from build123d import *

# Parameters (mm, degrees)
ESQUISSE1_R             = 38.5
BOSS_EXTRU_1_DEPTH      = 100
ENL_V_START             = -95
ESQUISSE2_R             = 38.5
ESQUISSE2_R_2           = 28.5
ENL_V_MAT_EXTRU_1_DEPTH = 95
ESQUISSE4_R             = 22.5
ENL_V_MAT_EXTRU_2_DEPTH = 45
ESQUISSE5_R             = 18.5
ENL_V_MAT_EXTRU_3_DEPTH = 9
ESQUISSE6_R             = 12
ENL_V_MAT_EXTRU_4_DEPTH = 77.684418235
D_GAGEMENT_M222_D       = 24
ESQUISSE14_R            = 1.5
ENL_V_MAT_EXTRU_8_DEPTH = 77.684418235
ENL_V_START_2           = -9
ESQUISSE16_R            = 18.5
ENL_V_MAT_EXTRU_9_DEPTH = 9


with BuildPart() as part:
    # Esquisse1 → Boss.-Extru.1 (new body)
    with BuildSketch(Plane(origin=(0, 0, 0), x_dir=(1, 0, 0), z_dir=(0, 1, 0))):
        with Locations(Location((0, 0, 0), (0, 0, 270))):
            Circle(ESQUISSE1_R)
    extrude(amount=BOSS_EXTRU_1_DEPTH)

    # Esquisse2 → Enlèv. mat.-Extru.1 (cut)
    with BuildSketch(Plane(origin=(0, 100, 0), x_dir=(1, 0, 0), z_dir=(0, 1, 0)).offset(ENL_V_START)):
        with Locations(Location((0, 0, 0), (0, 0, 270))):
            Circle(ESQUISSE2_R)
        with Locations(Location((0, 0, 0), (0, 0, 270))):
            Circle(ESQUISSE2_R_2, mode=Mode.SUBTRACT)
    extrude(amount=ENL_V_MAT_EXTRU_1_DEPTH, mode=Mode.SUBTRACT)

    # Esquisse4 → Enlèv. mat.-Extru.2 (cut)
    with BuildSketch(Plane(origin=(0, 0, 0), x_dir=(-1, 0, 0), z_dir=(0, -1, 0))):
        with Locations(Location((0, 0, 0), (0, 0, 90))):
            Circle(ESQUISSE4_R)
    extrude(amount=-ENL_V_MAT_EXTRU_2_DEPTH, mode=Mode.SUBTRACT)

    # Esquisse5 → Enlèv. mat.-Extru.3 (cut)
    with BuildSketch(Plane(origin=(0, 45, 0), x_dir=(-1, 0, 0), z_dir=(0, -1, 0))):
        with Locations(Location((0, 0, 0), (0, 0, 90))):
            Circle(ESQUISSE5_R)
    extrude(amount=-ENL_V_MAT_EXTRU_3_DEPTH, mode=Mode.SUBTRACT)

    # Esquisse6 → Enlèv. mat.-Extru.4 (cut, through all)
    with BuildSketch(Plane(origin=(0, 54, 0), x_dir=(-1, 0, 0), z_dir=(0, -1, 0))):
        with Locations(Location((0, 0, 0), (0, 0, 90))):
            Circle(ESQUISSE6_R)
    extrude(amount=-ENL_V_MAT_EXTRU_4_DEPTH, mode=Mode.SUBTRACT)

    # Dégagement M222 (through all)
    with Locations(Plane(origin=(0, 72.5, 28.5), x_dir=(1, 0, 0), z_dir=(0, 0, 1))):
        with Locations((0, 0)):
            Hole(D_GAGEMENT_M222_D / 2)

    # Esquisse14 → Enlèv. mat.-Extru.8 (cut, through all)
    with BuildSketch(Plane(origin=(0, 54, 0), x_dir=(-1, 0, 0), z_dir=(0, -1, 0))):
        with Locations(Location((0, -33.5, 0), (0, 0, 270))):
            Circle(ESQUISSE14_R)
        with Locations(Location((-29.011851027, -16.75, 0), (0, 0, 270))):
            Circle(ESQUISSE14_R)
        with Locations(Location((-29.011851027, 16.75, 0), (0, 0, 270))):
            Circle(ESQUISSE14_R)
        with Locations(Location((0, 33.5, 0), (0, 0, 270))):
            Circle(ESQUISSE14_R)
        with Locations(Location((29.011851027, 16.75, 0), (0, 0, 270))):
            Circle(ESQUISSE14_R)
        with Locations(Location((29.011851027, -16.75, 0), (0, 0, 270))):
            Circle(ESQUISSE14_R)
    extrude(amount=ENL_V_MAT_EXTRU_8_DEPTH, mode=Mode.SUBTRACT)

    # Esquisse16 → Enlèv. mat.-Extru.9 (cut)
    with BuildSketch(Plane(origin=(0, 100, 0), x_dir=(1, 0, 0), z_dir=(0, 1, 0)).offset(ENL_V_START_2)):
        with Locations(Location((0, 0, 0), (0, 0, 90))):
            Circle(ESQUISSE16_R)
    extrude(amount=ENL_V_MAT_EXTRU_9_DEPTH, mode=Mode.SUBTRACT)


solid = part.part
Here's how the part is built. I have some questions about the finished solid (model axes, mm). A direction names the side the tool comes from. Coordinates: 2 decimals unless noted, no trailing zeros. Order: outer loops, then holes, each group sorted by start corner. A loop starts at its lowest first (then second) coordinate and runs counter-clockwise, first axis right, second up. Notation, with made-up numbers: M -11,87 L -4,87 A9 cw -4,93 Z; hole C 79,-15.5 d4. An arc over 180 degrees is marked long. Answer as CSV lines item,"result". Start each with the question number.
1. For pin 1 (4 mm diameter, centred on x = 29.01, z = -16.75, fed in from -Y); pin 2 (1 mm diameter, centred on y = 32.5, z = 5, fed in from +X); pin 3 (3 mm diameter, centred on x = 22, y = 62, fed in from +Z); pin 4 (4 mm diameter, centred on y = 67, z = -9.5, fed in from -X), each with a flat end and sliding along its axis, tell me the tip position at first contact or that it passes through.
2. I want a section at C-C, the plane z = -6.5. Write out the boundary of the cut face in (x, y), and give its area (3 significant figures).
3. I want a section at A-A, the plane z = -16.75. Count the separate pieces of the cut face and the enclosed holes in it, and give its area (3 significant figures).
4. On a 3-axis mill with a long thin cutter (end or side, diameter ignored), from which of +Z, -Z, +X, -X, +Y, -Y can I reach the whole of each face in a straight line? I mean faces 5 (the flat face through (29, 5, 0)), 6 (the cylindrical face through (11.9, 85.73, 1.56)), 7 (the flat face through (-18, 45, 5)). Say none if no direction works.
5. We'd pull the mould along X, two halves only. Please class faces 1 (the cylindrical face through (7.086, 95.437, -17.089)), 2 (the cylindrical face through (-37.584, 2.465, -8.346)), 3 (the cylindrical face through (30.476, 2.535, -17.075)), 4 (the flat face through (-17, 0, 17)): released by +X, released by -X, zero draft, split by the parting line, or undercut.
6. I need wall thicknesses on line 1 (Y direction, x = -30.5, z = 5.5); line 2 (Y direction, x = -3, z = 18.5); line 3 (X direction, y = 54.5, z = -2.5). Which ranges of each line are inside material? Lowest first, please. Write a range as [from, to].
7. I want a section at B-B, the plane y = 64. Write out the boundary of the cut face in (x, z), and give its area (3 significant figures).
Recorded:
1,pin 1,"stops at y = 0"
1,pin 2,"stops at x = 28.14"
1,pin 3,"stops at z = 19.8"
1,pin 4,"stops at x = -27.5"
2,outline,"M -37.95,0 L -21.54,0 L -21.54,45 L -17.32,45 L -17.32,54 L -10.09,54 L -10.09,66 A12 cw -10.09,79 L -10.09,91 L -17.32,91 L -17.32,100 L -27.75,100 L -27.75,5 L -37.95,5 Z; M 10.09,54 L 17.32,54 L 17.32,45 L 21.54,45 L 21.54,0 L 37.95,0 L 37.95,5 L 27.75,5 L 27.75,100 L 17.32,100 L 17.32,91 L 10.09,91 L 10.09,79 A12 cw 10.09,66 Z"
2,area,"2,310 mm2"
3,separate pieces,"3"
3,enclosed holes,"1"
3,area,"2,610 mm2"
4,face 5,"+Y"
4,face 6,"+Y, -Y"
4,face 7,"-Y"
5,face 1,"undercut"
5,face 2,"split by the parting line"
5,face 3,"undercut"
5,face 4,"zero draft"
6,line 1,"y = [0, 5]"
6,line 2,"y = [45, 60.88], [84.12, 100]"
6,line 3,"x = [-28.39, -11.74], [11.74, 28.39]"
7,outline,"M -8.47,-27.21 L -8.47,-8.5 A12 cw -8.47,8.5 L -8.47,27.21 A28.5 ccw Z; M 8.47,-27.21 A28.5 ccw 8.47,27.21 L 8.47,8.5 A12 cw 8.47,-8.5 Z"
7,area,"1,520 mm2"
